Model file for the job. Use its own axes, mm. Round coordinates to 2 decimals unless told otherwise and drop trailing zeros. Answer in a Markdown table with one row per item.
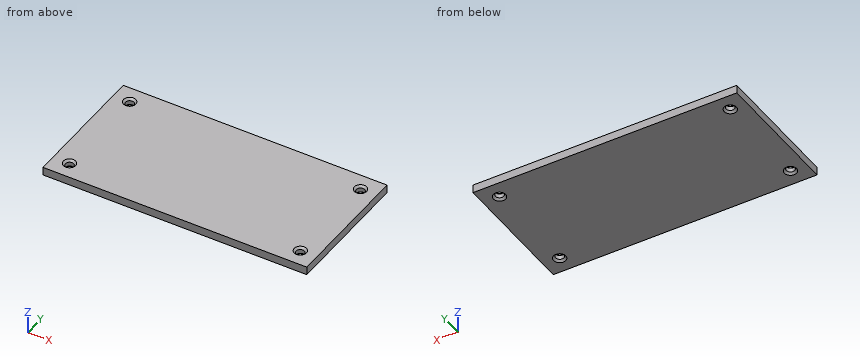
from build123d import *

# Parameters (mm, degrees)
F0_W     = 203.2
F0_H     = 101.6
F0_R     = 3.175
F1_DEPTH = 6.35
F2_SIZE2 = 1.5748
F2_SIZE  = 1.5748
F3_SIZE2 = 1.5748
F3_SIZE  = 1.5748


with BuildPart() as f1:
    # F0 (on Top) → F1 (new body)
    with BuildSketch(Plane.XY):
        with Locations((18.788079, 16.545452)):
            Rectangle(F0_W, F0_H)
        with Locations((-70.111921, -21.554548)):
            Circle(F0_R, mode=Mode.SUBTRACT)
        with Locations((107.688079, -21.554548)):
            Circle(F0_R, mode=Mode.SUBTRACT)
        with Locations((-70.111921, 54.645452)):
            Circle(F0_R, mode=Mode.SUBTRACT)
        with Locations((107.688079, 54.645452)):
            Circle(F0_R, mode=Mode.SUBTRACT)
    extrude(amount=F1_DEPTH)

    # F2
    f2_edges = [f1.edges().sort_by_distance(p)[0] for p in [
        (-66.936921, 54.645452, 3.175),
        (-73.286921, 54.645452, 0),
        (-73.286921, 54.645452, 6.35),
    ]]
    chamfer(f2_edges, length=F2_SIZE, length2=F2_SIZE2)

    # F3
    f3_edges = [f1.edges().sort_by_distance(p)[0] for p in [
        (110.863079, 54.645452, 3.175),
        (104.513079, 54.645452, 0),
        (104.513079, 54.645452, 6.35),
        (110.863079, -21.554548, 3.175),
        (104.513079, -21.554548, 0),
        (104.513079, -21.554548, 6.35),
        (-66.936921, -21.554548, 3.175),
        (-73.286921, -21.554548, 0),
        (-73.286921, -21.554548, 6.35),
    ]]
    chamfer(f3_edges, length=F3_SIZE, length2=F3_SIZE2)


solid = f1.part
1. Wall check: probe 1 along Y at (x, z) = (106, 0.75); probe 2 along X at (y, z) = (53.5, 3); probe 3 along X at (y, z) = (56, 4.5). Give the ranges that are in metal, low to high.
Verdict:
| item | result |
|---|---|
| probe 1 | y = -34.25 to -25.18, -17.93 to 51.02, 58.27 to 67.35 |
| probe 2 | x = -82.81 to -73.07, -67.15 to 104.73, 110.65 to 120.39 |
| probe 3 | x = -82.81 to -72.98, -67.24 to 104.82, 110.56 to 120.39 |
2. Pin check, flat tip, straight feed: pin 1 (10 mm diameter, centred on x = -70.11, y = -21.55, fed in from -Z). Stop position of the tip, or through.
Verdict:
| item | result |
|---|---|
| pin 1 | stops at z = 0 |
3. Saw through at A-A (x = -69). State how many separate pieces and enclosed holes the cut face has, and give its area (3 significant figures).
Verdict:
| item | result |
|---|---|
| separate pieces | 3 |
| enclosed holes | 0 |
| area | 559 mm² |
